Input: part model. Units: mm. Frame: model coordinates. A direction names the side the tool comes from. Give positions to 0.01 mm unless a question says otherwise; leave off trailing zeros. Loops run counter-clockwise (first coordinate to the right, second up) from the corner with the lowest first, then second, coordinate; pieces in that order, holes last. Notation, with made-up numbers: (35, 9.5) - (60, 9.5) arc R19 ccw to (60, 25.5) - close; hole circle Ø3 at (-36.5, 68). An arc over 180 degrees is marked (long way). Answer as a JSON object with one key per item and string values. Group by question number.
(1) Pin query (flat end, axial travel): P1, Ø1, axis at x = 32.5, z = -8, coming from the +Y side; P2, Ø1.6, axis at x = 13, z = -8, coming from the +Y side. Return the tip coordinate at first contact, or that it passes through.
(2) Material intervals for L1, parallel to X at y = 11.05, z = -10.5; L2, parallel to X at y = 10.9, z = -12.75, sorted ascending.
(3) Access query for faces 4 (the flat face through (23, 9, -5)), 5 (the flat face through (20, 12.252, -10)), 6 (the flat face through (23, 10.342, -10)), 7 (the flat face through (33, 10.342, -10)), 8 (the flat face through (13, 10.342, -10)). Directions: +Z, -Z, +X, -X, +Y, -Y. A direction counts if a zero-diameter tool reaches every point of the face in a straight line with its end or side. Return the directions, or none.
(4) Section query A-A (y = 11.85). Return loops of the section in (x, z), plus the area to 3 significant figures.
(5) Section query C-C (x = 17.25). Return loops of the section in (y, z), plus the area to 3 significant figures.
(6) Mould query, pull axis X, two halves, no side actions, for faces 1 (the cylindrical face through (13.96, 11.23, -9.93)), 2 (the cylindrical face through (21.03, 11.26, -9.93)), 3 (the flat face through (25, 12.252, -10)). Classes: +X half, -X half, draft (parallel to the pull), parting line (faces both ways), or undercut.
(7) Section query D-D (x = 21.25). Return loops of the section in (y, z).
(8) Section query B-B (z = -9). Return loops of the section in (x, y) (1 decimal).
Autodesk Inventor part; units mm, degrees
ref_plane "C1_XY" through (0, 0, 0) normal (0, 0, 1) x (1, 0, 0)
ref_plane "C1_YZ" through (0, 0, 0) normal (1, 0, 0) x (0, 1, 0)
ref_plane "C1_ZX" through (0, 0, 0) normal (0, 1, 0) x (0, 0, 1)
sketch "Sketch_1" plane through (0, 0, 0) normal (0, 0, 1) x (1, 0, 0)
  line L0 (10, 12.2524) -> (10.875, 12.2524)
  arc A0 (10.875, 12.2524) -> (11.4955, 10.3424) centre (14.125, 12.2524) ccw
  line L1 (11.4955, 10.3424) -> (13.5045, 10.3424)
  arc A1 (13.5045, 10.3424) -> (14.125, 12.2524) centre (10.875, 12.2524) ccw
  line L2 (14.125, 12.2524) -> (15.875, 12.2524)
  arc A2 (15.875, 12.2524) -> (16.4955, 10.3424) centre (19.125, 12.2524) ccw
  line L3 (16.4955, 10.3424) -> (18.5045, 10.3424)
  arc A3 (18.5045, 10.3424) -> (19.125, 12.2524) centre (15.875, 12.2524) ccw
  line L4 (19.125, 12.2524) -> (20.875, 12.2524)
  arc A4 (20.875, 12.2524) -> (21.4955, 10.3424) centre (24.125, 12.2524) ccw
  line L5 (21.4955, 10.3424) -> (23.5045, 10.3424)
  arc A5 (23.5045, 10.3424) -> (24.125, 12.2524) centre (20.875, 12.2524) ccw
  line L6 (24.125, 12.2524) -> (25.875, 12.2524)
  arc A6 (25.875, 12.2524) -> (26.4955, 10.3424) centre (29.125, 12.2524) ccw
  line L7 (26.4955, 10.3424) -> (28.5045, 10.3424)
  arc A7 (28.5045, 10.3424) -> (29.125, 12.2524) centre (25.875, 12.2524) ccw
  line L8 (29.125, 12.2524) -> (30.875, 12.2524)
  arc A8 (30.875, 12.2524) -> (31.4955, 10.3424) centre (34.125, 12.2524) ccw
  line L9 (31.4955, 10.3424) -> (33.5045, 10.3424)
  arc A9 (33.5045, 10.3424) -> (34.125, 12.2524) centre (30.875, 12.2524) ccw
  line L10 (34.125, 12.2524) -> (35, 12.2524)
  line L11 (35, 12.2524) -> (35, 13.7524)
  line L12 (35, 13.7524) -> (10, 13.7524)
  line L13 (10, 13.7524) -> (10, 12.2524)
extrude "Extrusion1" add sketch "Sketch_1" along normal mid plane 10
sketch "Sketch_2" plane through (0, 0, 0) normal (0, 0, 1) x (1, 0, 0)
  arc A0 (0, 13.7524) -> (0, -13.7524) centre (0, 0) ccw
  line L0 (0, -13.7524) -> (260, -13.7524)
  arc A1 (260, -13.7524) -> (260, 13.7524) centre (260, 0) ccw
  line L1 (260, 13.7524) -> (0, 13.7524)
  arc A2 (0, 12.2524) -> (0, -12.2524) centre (0, 0) ccw
  line L2 (0, -12.2524) -> (260, -12.2524)
  arc A3 (260, -12.2524) -> (260, 12.2524) centre (260, 0) ccw
  line L3 (260, 12.2524) -> (0, 12.2524)
extrude "Extrusion2" add sketch "Sketch_2" along normal mid plane 10
ref_plane "C1_XY" through (0, 0, 0) normal (0, 0, 1) x (1, 0, 0)
ref_plane "C1_YZ" through (0, 0, 0) normal (1, 0, 0) x (0, 1, 0)
ref_plane "C1_ZX" through (0, 0, 0) normal (0, 1, 0) x (0, 0, 1)
sketch "スケッチ3" plane through (0, 0, -5) normal (0, 0, -1) x (-1, 0, 0)
  line L0 (-33.5045, 12.2524) -> (-11.4955, 12.2524)
  line L1 (-11.4955, 12.2524) -> (-11.4955, 7.3424)
  line L2 (-11.4955, 7.3424) -> (-33.5045, 7.3424)
  line L3 (-33.5045, 7.3424) -> (-33.5045, 12.2524)
  line L4 (-33.5045, 10.3424) -> (-31.4955, 10.3424)
  line L5 (-30.71, 12.2524) -> (-29.125, 12.2524)
  arc A0 (-29.125, 12.2524) -> (-28.5045, 10.3424) centre (-25.875, 12.2524) ccw
  line L6 (-28.5045, 10.3424) -> (-26.4955, 10.3424)
  arc A1 (-26.4955, 10.3424) -> (-25.875, 12.2524) centre (-29.125, 12.2524) ccw
  line L7 (-25.875, 12.2524) -> (-24.125, 12.2524)
  arc A2 (-24.125, 12.2524) -> (-23.5045, 10.3424) centre (-20.875, 12.2524) ccw
  line L8 (-23.5045, 10.3424) -> (-21.4955, 10.3424)
  arc A3 (-21.4955, 10.3424) -> (-20.875, 12.2524) centre (-24.125, 12.2524) ccw
  line L9 (-20.875, 12.2524) -> (-19.125, 12.2524)
  arc A4 (-19.125, 12.2524) -> (-18.5045, 10.3424) centre (-15.875, 12.2524) ccw
  line L10 (-18.5045, 10.3424) -> (-16.4955, 10.3424)
  arc A5 (-16.4955, 10.3424) -> (-15.875, 12.2524) centre (-19.125, 12.2524) ccw
  line L11 (-15.875, 12.2524) -> (-14.125, 12.2524)
  line L12 (-13.5045, 10.3424) -> (-11.4955, 10.3424)
  arc A6 (-31.4955, 10.3424) -> (-30.875, 12.2524) centre (-34.125, 12.2524) ccw
  arc A7 (-34.125, 12.2524) -> (-33.5045, 10.3424) centre (-30.875, 12.2524) ccw
  arc A8 (-14.125, 12.2524) -> (-13.5045, 10.3424) centre (-10.875, 12.2524) ccw
  arc A9 (-11.4955, 10.3424) -> (-10.875, 12.2524) centre (-14.125, 12.2524) ccw
  point P0 (0, 0)
  point P1 (-30.71, 12.2472)
  point P2 (-15.875, 12.2524)
  point P3 (-20.875, 12.2524)
  point P4 (-25.875, 12.2524)
  point P5 (-30.875, 12.2524)
  dimension "d4" = 3
extrude "押し出し3" add sketch "スケッチ3" along normal blind 10 contours L0 A0 L6 A1 A2 L8 A3 A4 L10 A5 A8 L12 L1 L2 L3 L4 A6
sketch "スケッチ4" plane through (0, 13.7524, 5) normal (0, 1, 0) x (1, 0, 0)
  line L0 (-13.7524, 0) -> (0, 0)
  line L1 (273.7524, 10) -> (260, 10)
  line L2 (-13.7524, 0) -> (273.7524, 0)
  line L3 (273.7524, 0) -> (273.7524, 10)
  line L4 (273.7524, 10) -> (-13.7524, 10)
  line L5 (-13.7524, 10) -> (-13.7524, 0)
  point P0 (0, 5)
extrude "押し出し4" cut sketch "スケッチ4" against normal through all
properties part number "HTBN600S5M-100_info-1-16-16" material "ABS プラスチック"
Recorded:
{
 "1": {"P1": "stops at y = 10.34", "P2": "stops at y = 10.84"},
 "2": {"L1": "x = 13.89 to 16.11, 18.89 to 21.11, 23.89 to 26.11, 28.89 to 31.11", "L2": "x = 13.83 to 16.17, 18.83 to 21.17, 23.83 to 26.17, 28.83 to 31.17"},
 "3": {"face 4": "+Z, +X, -X, +Y, -Y", "face 5": "+Z, -Z, +X, -X, +Y", "face 6": "+Z, -Z, +Y", "face 7": "+Z, -Z, +X, +Y", "face 8": "+Z, -Z, -X, +Y"},
 "4": {"outline": "(14.1, -15) - (15.9, -15) - (15.9, -5) - (14.1, -5) - close; (19.1, -15) - (20.9, -15) - (20.9, -5) - (19.1, -5) - close; (24.1, -15) - (25.9, -15) - (25.9, -5) - (24.1, -5) - close; (29.1, -15) - (30.9, -15) - (30.9, -5) - (29.1, -5) - close", "area": "72.0 mm^2"},
 "5": {"outline": "(7.34, -15) - (10.34, -15) - (10.34, -5) - (7.34, -5) - close", "area": "30.0 mm^2"},
 "6": {"face 1": "-X half", "face 2": "undercut", "face 3": "draft"},
 "7": {"outline": "(7.34, -15) - (10.74, -15) - (10.74, -5) - (7.34, -5) - close"},
 "8": {"outline": "(11.5, 7.3) - (33.5, 7.3) - (33.5, 10.3) - (31.5, 10.3) arc R3.3 cw to (30.9, 12.3) - (29.1, 12.3) arc R3.2 cw to (28.5, 10.3) - (26.5, 10.3) arc R3.3 cw to (25.9, 12.3) - (24.1, 12.3) arc R3.2 cw to (23.5, 10.3) - (21.5, 10.3) arc R3.3 cw to (20.9, 12.3) - (19.1, 12.3) arc R3.2 cw to (18.5, 10.3) - (16.5, 10.3) arc R3.3 cw to (15.9, 12.3) - (14.1, 12.3) arc R3.2 cw to (13.5, 10.3) - (11.5, 10.3) - close"}
}
